```python
from build123d import *

# Parameters (mm, degrees)
CROQUIS1_R              = 13.4
CROQUIS1_R_2            = 10.65
SALIENTE_EXTRUIR1_DEPTH = 25.4
CROQUIS2_R              = 44
CROQUIS2_R_2            = 10.65
CROQUIS2_R_3            = 3
SALIENTE_EXTRUIR2_DEPTH = 3.4


with BuildPart() as part:
    # Croquis1 → Saliente-Extruir1 (new body)
    with BuildSketch(Plane.XY):
        Circle(CROQUIS1_R)
        Circle(CROQUIS1_R_2, mode=Mode.SUBTRACT)
    extrude(amount=SALIENTE_EXTRUIR1_DEPTH)

    # Croquis2 → Saliente-Extruir2 (add)
    with BuildSketch(Plane.XY.offset(25.4)):
        Circle(CROQUIS2_R)
        Circle(CROQUIS2_R_2, mode=Mode.SUBTRACT)
        with Locations((0, 30)):
            Circle(CROQUIS2_R_3, mode=Mode.SUBTRACT)
        with Locations((25.980762114, 15)):
            Circle(CROQUIS2_R_3, mode=Mode.SUBTRACT)
        with Locations((25.980762114, -15)):
            Circle(CROQUIS2_R_3, mode=Mode.SUBTRACT)
        with Locations((0, -30)):
            Circle(CROQUIS2_R_3, mode=Mode.SUBTRACT)
        with Locations((-25.980762114, -15)):
            Circle(CROQUIS2_R_3, mode=Mode.SUBTRACT)
        with Locations((-25.980762114, 15)):
            Circle(CROQUIS2_R_3, mode=Mode.SUBTRACT)
    extrude(amount=SALIENTE_EXTRUIR2_DEPTH)


solid = part.part
```
The model under review builds one solid part; all positions refer to its coordinate system, in mm. A direction names the side the tool comes from. Coordinates: 2 decimals unless noted, no trailing zeros. Order: outer loops, then holes, each group sorted by start corner. A loop starts at its lowest first (then second) coordinate and runs counter-clockwise, first axis right, second up. Notation, with made-up numbers: (-36, 66) -> (-22, 66) arc R27 cw to (-22, 102) -> close; hole circle Ø2 at (-32.5, 84). An arc over 180 degrees is marked (long way). Answer in a Markdown table with one row per item. Add a question column.
Item 1: We need section A-A on x = 0. Write out the cut boundary in (y, z), plus the area to 3 significant figures.
Item 2: We need section D-D on z = 11.25. Write out the cut boundary in (x, y), plus the area to 3 significant figures.
Item 3: We need section B-B on y = 0. Write out the cut boundary in (x, z).
Item 4: Mouldability with a two-part tool opening along Y and no side actions: class faces 1 (the flat face through (-10.4, -9.2, 25.4)), 2 (the cylindrical face through (-9.538, -42.954, 27.076)), 3 (the cylindrical face through (27.37, -17.66, 27.08)) as +Y half, -Y half, draft (parallel to the pull), parting line (faces both ways), or undercut.
Item 5: Machinability: for faces 4 (the cylindrical face through (27.37, 12.34, 27.08)), 5 (the cylindrical face through (-13.387, 0.589, 12.522)), which of the approach directions +Z, -Z, +X, -X, +Y, -Y give a long, thin tool a straight path to every point of the face, cutting with its end or side? Answer none if there is none.
Item 6: We need section C-C on y = 15. Write out the cut boundary in (x, z), plus the area to 3 significant figures.
Item 7: To check wall thickness, follow probe 1 along Y at (x, z) = (0, 27.45); probe 2 along Z at (x, y) = (15.5, -32.5); probe 3 along X at (y, z) = (-1, 16). State the ranges of each line that lie inside material, in increasing order.
Item 8: Clearance check with flat-ended pins moving along their axes: pin 1 (3 mm diameter, centred on x = 9.5, z = 12.5, fed in from +Y); pin 2 (1 mm diameter, centred on x = 26, y = -33.5, fed in from -Z); pin 3 (10 mm diameter, centred on y = 2, z = 18.5, fed in from +X). State where each tip first meets the part, or that it passes through.
Final values:
| question | item | result |
|---|---|---|
| 1 | outline | (-44, 25.4) -> (-33, 25.4) -> (-33, 28.8) -> (-44, 28.8) -> close; (-27, 25.4) -> (-13.4, 25.4) -> (-13.4, 0) -> (-10.65, 0) -> (-10.65, 28.8) -> (-27, 28.8) -> close; (10.65, 0) -> (13.4, 0) -> (13.4, 25.4) -> (27, 25.4) -> (27, 28.8) -> (10.65, 28.8) -> close; (33, 25.4) -> (44, 25.4) -> (44, 28.8) -> (33, 28.8) -> close |
| 1 | area | 326 mm2 |
| 2 | outline | circle Ø26.8 at (0, 0); hole circle Ø21.3 at (0, 0) |
| 2 | area | 208 mm2 |
| 3 | outline | (-44, 25.4) -> (-13.4, 25.4) -> (-13.4, 0) -> (-10.65, 0) -> (-10.65, 28.8) -> (-44, 28.8) -> close; (10.65, 0) -> (13.4, 0) -> (13.4, 25.4) -> (44, 25.4) -> (44, 28.8) -> (10.65, 28.8) -> close |
| 4 | face 1 | draft |
| 4 | face 2 | parting line |
| 4 | face 3 | undercut |
| 5 | face 4 | +Z, -Z |
| 5 | face 5 | -Z |
| 6 | outline | (-41.36, 25.4) -> (-28.98, 25.4) -> (-28.98, 28.8) -> (-41.36, 28.8) -> close; (-22.98, 25.4) -> (22.98, 25.4) -> (22.98, 28.8) -> (-22.98, 28.8) -> close; (28.98, 25.4) -> (41.36, 25.4) -> (41.36, 28.8) -> (28.98, 28.8) -> close |
| 6 | area | 240 mm2 |
| 7 | probe 1 | y = -44 to -33, -27 to -10.65, 10.65 to 27, 33 to 44 |
| 7 | probe 2 | z = 25.4 to 28.8 |
| 7 | probe 3 | x = -13.36 to -10.6, 10.6 to 13.36 |
| 8 | pin 1 | stops at y = 10.75 |
| 8 | pin 2 | stops at z = 25.4 |
| 8 | pin 3 | stops at x = 13.4 |
